CAD build for the part. Positions are in the model's coordinates, mm. A direction names the side the tool comes from. Give positions to 0.01 mm unless a question says otherwise; leave off trailing zeros.
Item 1: Flat gauge pins, fed straight in: P1, Ø1, axis at x = 10, z = 138, coming from the -Y side; P2, Ø3, axis at y = -60.5, z = -98, coming from the -X side; P3, Ø1, axis at x = 7, z = -314, coming from the -Y side; P4, Ø5, axis at x = 7.5, z = 193.5, coming from the -Y side. Where does each tip first touch, or does it go through?
Item 2: Wall check: L1, parallel to Y at x = 16.5, z = -252; L2, parallel to Y at x = 3.75, z = 135. Give the ranges that are in metal, low to high.
Item 3: Which spindle directions (+Z, -Z, +X, -X, +Y, -Y) get a long thin tool onto all of the face, cutting with end or side? Do faces 1 (the flat face through (9.126, -288.216, 405.42)), 2 (the flat face through (18, -1, 6)). Say none if no direction does.
```python
from build123d import *

# Parameters (mm, degrees)
F0_W     = 622
F0_H     = 870
F1_DEPTH = 18
F3_DEPTH = 870
F5_DEPTH = 60


with BuildPart() as f1:
    # F0 (on Right) → F1 (new body)
    with BuildSketch(Plane.YZ):
        Rectangle(F0_W, F0_H)
    extrude(amount=F1_DEPTH)

    # F2 (on face) → F3 (cut)
    with BuildSketch(Plane.XY.offset(435)):
        Polygon((0, 304.090447), (18, 311), (0, 311), align=None)
        Polygon((18, -304.090447), (0, -311), (18, -311), align=None)
    extrude(amount=-F3_DEPTH, mode=Mode.SUBTRACT)

    # F4 (on face) → F5 (cut)
    with BuildSketch(Plane.XY.offset(435)):
        Polygon((0, -291.71939), (0, -311), (18, -304.090447), (18, -284.809837), align=None)
    extrude(amount=-F5_DEPTH, mode=Mode.SUBTRACT)


solid = f1.part
```
The answers:
1. P1: stops at y = -307.35
1. P2: stops at x = 0
1. P3: stops at y = -308.5
1. P4: stops at y = -309.08
2. L1: y = -304.67 to 310.42
2. L2: y = -309.56 to 305.53
3. face 1: +Z, +X, -Y
3. face 2: +Z, -Z, +X, +Y, -Y
